Part model, mm, in its own coordinate system. Face numbers are marked on the shaded views. A direction names the side the tool comes from. Round coordinates to 2 decimals unless told otherwise and drop trailing zeros. Loops run counter-clockwise (first coordinate to the right, second up) from the corner with the lowest first, then second, coordinate; pieces in that order, holes last.
(1) Probe probe 1 along X at (y, z) = (210.75, 12.2); probe 2 along Y at (x, z) = (-247.75, 13.4); probe 3 along Z at (x, y) = (-250.9, 210.5). List the from-to ranges inside material, lowest first.
(2) Cut at D-D on x = -253.75. List the corners of the cut face in (y, z).
(3) Mould opens along X. For the marked faces 4, 5, 6 and 7 say: +X half, -X half, draft (parallel to the pull), parting line (faces both ways), or undercut.
(4) Cut at C-C on y = 210. List the corners of the cut face in (x, z).
(5) Cut at A-A on y = 224. List the corners of the cut face in (x, z), then the cut area to 3 significant figures.
(6) Flat gauge pins, fed straight in: pin 1 (0.8 mm diameter, centred on x = -240.5, z = 13, fed in from +Y); pin 2 (1.5 mm diameter, centred on x = -246.5, y = 216.5, fed in from +Z); pin 3 (0.6 mm diameter, centred on x = -243, z = 12, fed in from -Y). Where does each tip first touch, or does it go through?
(7) Tool access for the marked faces 1, 2 and 3: list every direction of +Z, -Z, +X, -X, +Y, -Y with a clear straight run to the whole face (end or side of a thin tool).
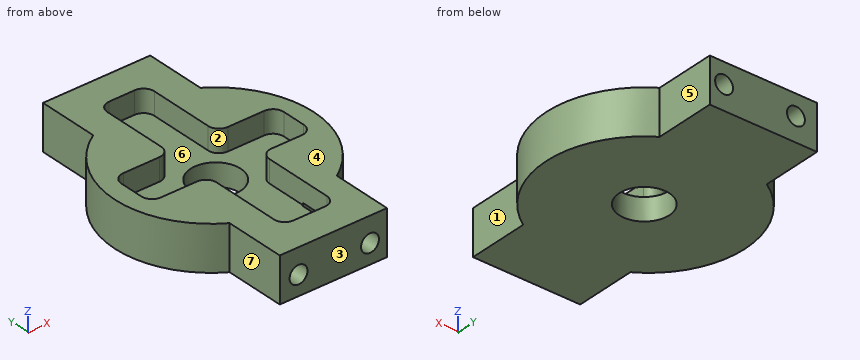
from build123d import *

# Parameters (mm, degrees)
SKETCH1_R           = 2.8
BOSS_EXTRUDE1_DEPTH = 5
CUT_EXTRUDE1_DEPTH  = 2.5
FILLET1_R           = 1.2
SKETCH3_R           = 1
CUT_EXTRUDE2_DEPTH  = 8
SKETCH4_R           = 1
CUT_EXTRUDE3_DEPTH  = 8


with BuildPart() as part:
    # Sketch1 → Boss-Extrude1 (new body)
    with BuildSketch(Plane.XY.offset(10)):
        with BuildLine():
            Line((-253, 240), (-241, 240))
            Line((-241, 240), (-241, 233.219543457))
            ThreePointArc((-241, 233.219543457), (-235.964643127, 224), (-241, 214.780456543))
            Line((-241, 214.780456543), (-241, 208))
            Line((-241, 208), (-253, 208))
            Line((-253, 208), (-253, 214.780456543))
            ThreePointArc((-253, 214.780456543), (-258.20228405, 224), (-253, 233.219543457))
            Line((-253, 233.219543457), (-253, 240))
        make_face()
        with Locations((-246.922635101, 224)):
            Circle(SKETCH1_R, mode=Mode.SUBTRACT)
    extrude(amount=BOSS_EXTRUDE1_DEPTH)

    # Sketch2 → Cut-Extrude1 (cut)
    with BuildSketch(Plane.XY.offset(15)):
        Polygon((-249.671711, 236.526764937), (-244.414971283, 236.526764937), (-244.414971283, 226.843297037), (-237.940881316, 226.843297037), (-237.940881316, 221.752559627), (-243.750962055, 221.752559627), (-243.750962055, 211.604094919), (-249.671711, 211.604094919), (-249.671711, 221.752559627), (-256.108895334, 221.752559627), (-256.108895334, 226.843297037), (-249.671711, 226.843297037), align=None)
    extrude(amount=-CUT_EXTRUDE1_DEPTH, mode=Mode.SUBTRACT)

    # Fillet1
    fillet1_edges = [part.edges().sort_by_distance(p)[0] for p in [
        (-249.671711, 226.843297037, 13.75),
        (-249.671711, 236.526764937, 13.75),
        (-244.414971283, 236.526764937, 13.75),
        (-244.414971283, 226.843297037, 13.75),
        (-237.940881316, 226.843297037, 13.75),
        (-237.940881316, 221.752559627, 13.75),
        (-243.750962055, 221.752559627, 13.75),
        (-243.750962055, 211.604094919, 13.75),
        (-249.671711, 211.604094919, 13.75),
        (-249.671711, 221.752559627, 13.75),
        (-256.108895334, 221.752559627, 13.75),
        (-256.108895334, 226.843297037, 13.75),
    ]]
    fillet(fillet1_edges, radius=FILLET1_R)

    # Sketch3 → Cut-Extrude2 (cut)
    with BuildSketch(Plane(origin=(0, 208, 0), x_dir=(-1, 0, 0), z_dir=(0, -1, 0))):
        with Locations(Location((250.9, -12.2, 0), (0, 0, 90))):
            Circle(SKETCH3_R)
        with Locations(Location((242.9, -12.2, 0), (0, 0, 90))):
            Circle(SKETCH3_R)
    extrude(amount=-CUT_EXTRUDE2_DEPTH, mode=Mode.SUBTRACT)

    # Sketch4 → Cut-Extrude3 (cut)
    with BuildSketch(Plane(origin=(0, 240, 0), x_dir=(1, 0, 0), z_dir=(0, 1, 0))):
        with Locations(Location((-242.598801613, -12.694978247, 0), (0, 0, 270))):
            Circle(SKETCH4_R)
        with Locations(Location((-250.64051394, -12.694978247, 0), (0, 0, 270))):
            Circle(SKETCH4_R)
    extrude(amount=-CUT_EXTRUDE3_DEPTH, mode=Mode.SUBTRACT)


solid = part.part
Final values:
1. probe 1: x = -253 to -251.9, -249.9 to -243.9, -241.9 to -241
1. probe 2: y = 208 to 211.6, 236.53 to 240
1. probe 3: z = 10 to 11.2, 13.2 to 15
2. outline: (215.28, 10) - (232.72, 10) - (232.72, 15) - (226.84, 15) - (226.84, 12.5) - (221.75, 12.5) - (221.75, 15) - (215.28, 15) - close
3. face 4: draft
3. face 5: +X half
3. face 6: undercut
3. face 7: -X half
4. outline: (-253, 10) - (-241, 10) - (-241, 15) - (-253, 15) - close; hole circle Ø2 at (-250.9, 12.2); hole circle Ø2 at (-242.9, 12.2)
5. outline: (-258.2, 10) - (-249.72, 10) - (-249.72, 12.5) - (-256.11, 12.5) - (-256.11, 15) - (-258.2, 15) - close; (-244.12, 10) - (-235.96, 10) - (-235.96, 15) - (-237.94, 15) - (-237.94, 12.5) - (-244.12, 12.5) - close
5. area: 51.8 mm2
6. pin 1: stops at y = 233.15
6. pin 2: stops at z = 12.5
6. pin 3: stops at y = 216
7. face 1: +Z, -Z, +X, -Y
7. face 2: +Z
7. face 3: +Z, -Z, +X, -X, -Y
